For this review, take the finished solid that the model builds, in its own axes (mm). A direction names the side the tool comes from. Give positions to 0.01 mm unless a question says otherwise; leave off trailing zeros. Loops run counter-clockwise (first coordinate to the right, second up) from the corner with the lowest first, then second, coordinate; pieces in that order, holes last. Notation, with made-up numbers: (37.25, -18) -> (80.25, -18) arc R29 cw to (80.25, 6) -> close; hole circle Ø4 at (19.25, 83). An arc over 180 degrees is marked (long way). Answer as CSV lines item,"result". Start each with the question number.
Item 1: Add section B-B on x = -121. State the section outline as (y, z) points.
Item 2: The part is to be moulded in two halves that separate along Z. For faces 1 (the face through (-117, 198, -35)), 2 (the face through (-119, 189, -64.914)), 3 (the face through (-120.621, 190.395, -19.316)), 4 (the face through (-105.081, 188.726, -41.13)), say which applies: +Z half, -Z half, draft (parallel to the pull), parting line (faces both ways), or undercut.
Item 3: Add section A-A on y = 196. State the section outline as (x, z) points, plus the area to 3 significant figures.
Item 4: Machinability: for faces 5 (the face through (-90.87, 190.39, -57.55)), 6 (the face through (-147.094, 190, -67)), 7 (the face through (-138.017, 188.726, -67.449)), 8 (the face through (-97.268, 190.395, -46.154)), which of the approach directions +Z, -Z, +X, -X, +Y, -Y give a long, thin tool a straight path to every point of the face, cutting with its end or side? Answer none if there is none.
Item 5: For L1, parallel to Z at x = -94, y = 191; L2, parallel to Z at x = -87.5, y = 196.75; L3, parallel to Z at x = -97.5, y = 191.75, list the stretches that pass through material, from the lowest coordinate up. Write a range as from..to.
Item 6: Clearance check with flat-ended pins moving along their axes: P1, Ø1.5, axis at y = 188, z = -49.5, coming from the +X side; P2, Ø3, axis at y = 194.5, z = -57, coming from the +X side; P3, Ø0.7, axis at x = -86, y = 192, coming from the +Z side; P4, Ø8, axis at x = -119, z = -13, coming from the -Y side. State where each tip first meets the part, or that it passes through.
Item 7: Add section D-D on x = -84. State the section outline as (y, z) points, plus the area to 3 significant figures.
Item 8: Add section C-C on x = -97.5. State the section outline as (y, z) points.
Autodesk Inventor part; units mm, degrees
ref_plane "YZ Plane" through (0, 0, 0) normal (1, 0, 0) x (0, 1, 0)
ref_plane "XZ Plane" through (0, 0, 0) normal (0, 1, 0) x (-1, 0, 0)
ref_plane "XY Plane" through (0, 0, 0) normal (0, 0, 1) x (1, 0, 0)
sketch "Sketch1" plane through (475.3607, 0, -304.7358) normal (0, 1, 0) x (-1, 0, 0)
  line L0 (-230.3144, -553.6037) -> (1418.8804, 1095.5912)
  line L1 (1257.2358, 1257.2358) -> (0, 0)
  line L2 (0, 0) -> (143.6839, -143.6842)
  line L3 (1418.8804, 1095.5912) -> (1257.2358, 1257.2358)
  line L4 (143.684, -143.6842) -> (-233.396, -520.7642)
  line L5 (-338.0775, -553.6037) -> (107.7631, -107.763)
  line L6 (89.8025, -89.8027) -> (-468.1591, -647.7642)
  line L7 (-468.1591, -647.7642) -> (1309.841, -647.7642)
  line L8 (1309.841, -520.7642) -> (-161.5539, -520.7642)
  line L9 (-161.5539, -520.7642) -> (-212.3539, -571.5642)
  line L10 (-212.3539, -571.5642) -> (-230.3144, -553.6037)
  line L11 (-233.396, -520.7642) -> (-269.317, -520.7642)
  line L12 (-269.317, -520.7642) -> (-320.117, -571.5642)
  line L13 (-320.117, -571.5642) -> (-338.0775, -553.6037)
  line L14 (1309.841, -647.7642) -> (1309.841, -520.7642)
  line L15 (107.7631, -107.763) -> (143.684, -143.6842)
  line L16 (143.6839, -143.6842) -> (-233.396, -520.7642)
  line L17 (-233.396, -520.7642) -> (-269.317, -520.7642)
  line L18 (-269.317, -520.7642) -> (-320.117, -571.5642)
  line L19 (-320.117, -571.5642) -> (-338.0775, -553.6037)
  line L20 (-338.0775, -553.6037) -> (107.7629, -107.7632)
extrude "Extrusion1" add sketch "Sketch1" along normal blind 381
sketch "Sketch2" plane through (943.5197, 0, -952.5) normal (0, 0, -1) x (-1, 0, 0)
  circle A0 centre (1524, 190.5) radius 50.8
  circle A1 centre (1016, 190.5) radius 50.8
  line L0 (1778, 0) -> (1778, 381)
  line L1 (0, 381) -> (1778, 381)
  point P0 (0, -381)
  dimension "d6" = 101.6
  dimension "d3" = 101.6
  dimension "d5" = 508
  dimension "d4" = 0
  dimension "d8" = 254
  dimension "d7" = 190.5
extrude "Extrusion2" cut sketch "Sketch2" against normal up to surface (127 mm away)
scale "Scale1" factors (0.03937, 0.03937, 0.03937) then translate (-114.2403, 183, -32.4136) bodies 1
sketch "Sketch3" plane through (-95.5254, 183, -44.4111) normal (0.7071068, 0, 0.7071068) x (0.7071068, 0, -0.7071068)
  circle A0 centre (-59.9999, 7.5) radius 2
  circle A1 centre (-9.9999, 7.5) radius 2
  line L0 (-69.9999, 15) -> (0, 15)
  line L1 (-69.9999, 0) -> (-69.9999, 15)
  point P0 (36.1433, -183)
  dimension "d15" = 4
  dimension "d16" = 4
  dimension "d17" = 7.5
  dimension "d18" = 0
  dimension "d19" = 50
  dimension "d20" = 10
extrude "Extrusion3" cut sketch "Sketch3" against normal blind 10
properties part number "charge" material "ABS Plastic"
Computed values:
1,outline,"(183, -69.91) -> (198, -69.91) -> (198, -64.91) -> (183, -64.91) -> close; (183, -31.66) -> (198, -31.66) -> (198, -18.94) -> (183, -18.94) -> close"
2,face 1,"draft"
2,face 2,"undercut"
2,face 3,"+Z half"
2,face 4,"undercut"
3,outline,"(-151.39, -1.28) -> (-86.46, -66.21) -> (-87.16, -66.91) -> (-89.16, -64.91) -> (-147.09, -64.91) -> (-147.09, -69.91) -> (-77.09, -69.91) -> (-99.06, -47.95) -> (-95.53, -44.41) -> (-145.02, 5.09) -> close; hole (-101.18, -50.07) -> (-86.34, -64.91) -> (-84.92, -64.91) -> (-82.92, -66.91) -> (-82.22, -66.21) -> (-99.77, -48.65) -> close"
3,area,"1,010 mm²"
4,face 5,"+Y, -Y"
4,face 6,"-Z, -X, +Y, -Y"
4,face 7,"-Z"
4,face 8,"+X, +Y, -Y"
5,L1,"-69.91..-64.91, -58.66..-57.25, -54.42..-53.01"
5,L2,"-69.91..-66.58, -65.16..-63.75, -60.92..-59.51"
5,L3,"-69.91..-64.91, -55.16..-53.75, -50.92..-49.51, -46.39..-42.44"
6,P1,"x = -96.76"
6,P2,"x = -88.51"
6,P3,"z = -60.66"
6,P4,"through"
7,outline,"(183, -69.91) -> (198, -69.91) -> (198, -65.84) -> (183, -65.84) -> close; (183, -64.42) -> (198, -64.42) -> (198, -63.01) -> (183, -63.01) -> close"
7,area,"82.4 mm²"
8,outline,"(183, -69.91) -> (198, -69.91) -> (198, -64.91) -> (183, -64.91) -> close; (183, -55.16) -> (198, -55.16) -> (198, -53.75) -> (183, -53.75) -> close; (183, -50.92) -> (198, -50.92) -> (198, -49.51) -> (183, -49.51) -> close; (183, -46.39) -> (198, -46.39) -> (198, -42.44) -> (183, -42.44) -> close"
